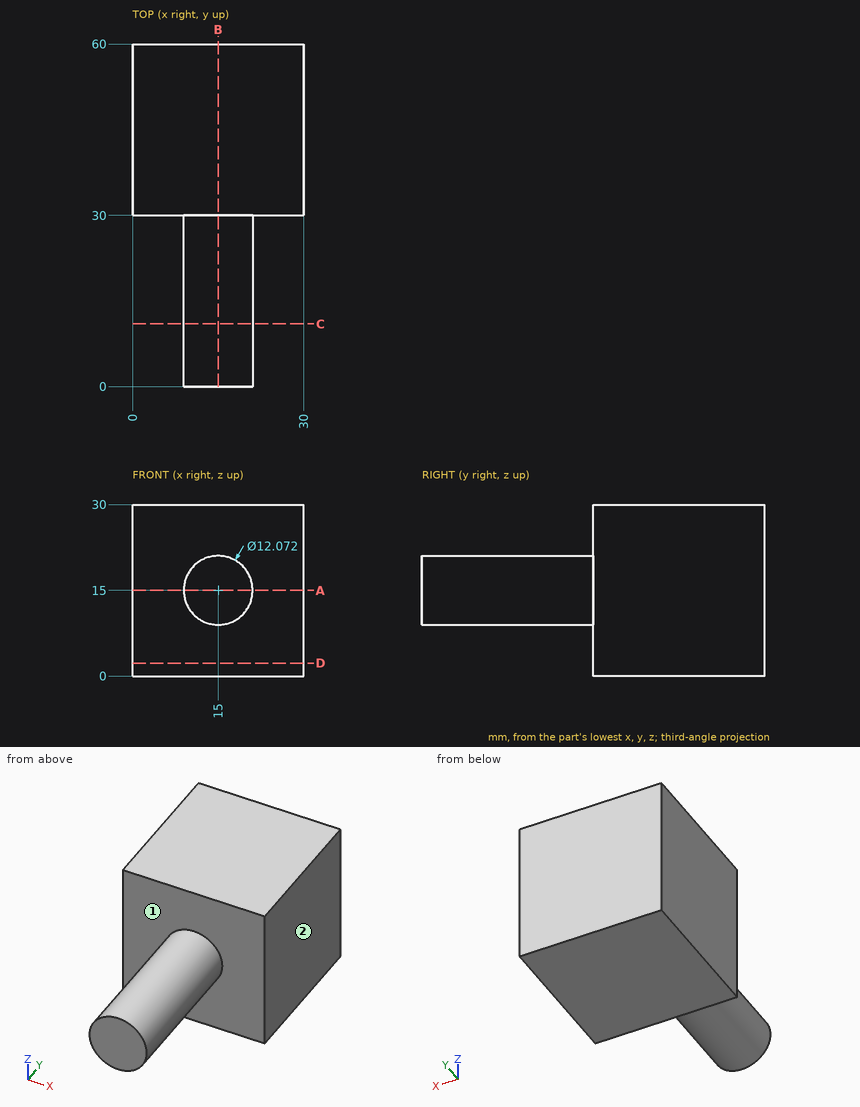
Part print with two shaded views. Sizes in mm from the minimum x, y, z corner. A direction names the side the tool comes from. Coordinates: 2 decimals unless noted, no trailing zeros. Write each loop counter-clockwise with the first axis right and the second up, starting at its lowest first coordinate (ties: lowest second). Pieces come first, ordered by that corner, then holes. Notation, with made-up numbers: (9, 27.25) -> (46, 27.25) arc R29 ccw to (46, 47.25) -> close; hole circle Ø4 at (24, 0). An arc over 180 degrees is marked (long way). Return JSON: item names as keys, results as strings. Group by question number.
Q1. Drill centre lines: line 1 (Y direction, x = 27, z = 1.5); line 2 (X direction, y = 7, z = 16); line 3 (X direction, y = 9, z = 20). Where is each one in solid material? Low to high.
Q2. Which spindle directions (+Z, -Z, +X, -X, +Y, -Y) get a long thin tool onto all of the face, cutting with end or side? Do the marked faces 1 and 2. Say none if no direction does.
Q3. Cut at C-C, the plane y = 11. Give the cut face in (x, z).
Q4. Cut at D-D, the plane z = 2.25. Give the cut face in (x, y), then the cut area to 3 significant figures.
Q5. Cut at B-B, the plane x = 15. Give the cut face in (y, z).
Q6. Cut at A-A, the plane z = 15. Give the cut face in (x, y), then the cut area to 3 significant figures.
Q7. Flat gauge pins, fed straight in: pin 1 (5 mm diameter, centred on x = 21.5, y = 14, fed in from -Z); pin 2 (6 mm diameter, centred on x = 19.5, z = 14.5, fed in from -Y). Where does each tip first touch, or does it go through?
Returned:
{
 "1": {"line 1": "y = 30 to 60", "line 2": "x = 9.05 to 20.95", "line 3": "x = 11.62 to 18.38"},
 "2": {"face 1": "-Y", "face 2": "+Z, -Z, +X, +Y, -Y"},
 "3": {"outline": "circle Ø12.07 at (15, 15)"},
 "4": {"outline": "(0, 30) -> (30, 30) -> (30, 60) -> (0, 60) -> close", "area": "900 mm2"},
 "5": {"outline": "(0, 8.96) -> (30, 8.96) -> (30, 0) -> (60, 0) -> (60, 30) -> (30, 30) -> (30, 21.04) -> (0, 21.04) -> close"},
 "6": {"outline": "(0, 30) -> (8.96, 30) -> (8.96, 0) -> (21.04, 0) -> (21.04, 30) -> (30, 30) -> (30, 60) -> (0, 60) -> close", "area": "1,260 mm2"},
 "7": {"pin 1": "stops at z = 10.48", "pin 2": "stops at y = 0"}
}
